Build history of the part. All positions in model axes, mm. Round coordinates to 2 decimals unless told otherwise and drop trailing zeros. Loops run counter-clockwise (first coordinate to the right, second up) from the corner with the lowest first, then second, coordinate; pieces in that order, holes last. Notation, with made-up numbers: (-32.5, 81.5) -> (-14.5, 81.5) arc R22 cw to (-14.5, 104.5) -> close; hole circle Ø7 at (-13.75, 78.25). An arc over 180 degrees is marked (long way). Put each result on its own line as item: value. Start each with the question number.
Item 1: Cut at A-A, the plane y = 4.5. List the corners of the cut face in (x, z).
Item 2: Cut at B-B, the plane z = 0. List the corners of the cut face in (x, y), plus the area to 3 significant figures.
Item 3: Drill centre lines: probe 1 along Z at (x, y) = (-2.5, 3.75); probe 2 along Z at (x, y) = (0, 2.5); probe 3 along X at (y, z) = (6.5, 1). Where is each one in solid material? Low to high. Write a range as [from, to].
Item 4: Cut at C-C, the plane x = 0. List the corners of the cut face in (y, z).
Item 5: Flat gauge pins, fed straight in: pin 1 Ø5.5 at (x, z) = (0, 0) entering from +Y; pin 2 Ø3 at (x, y) = (-1, 4) entering from +Z; pin 3 Ø3 at (x, y) = (-24, 1.5) entering from +Z; pin 4 Ø1 at (x, y) = (29, 7) entering from -Z. Where does each tip first touch, or does it go through?
Item 6: Pull direction Z, two halves, no side cores. Call faces 1 (the cylindrical face through (-1.73, 5.22, -7.81)), 2 (the flat face through (-1, 8, 9)), 3 (the conical face through (27.85, 0.14, -28.21)), 4 (the flat face through (3.4, 3, -3.4)): +Z half, -Z half, draft (parallel to the pull), parting line (faces both ways), or undercut.
```python
from build123d import *

# Parameters (mm, degrees)
F0_R     = 8
F1_DEPTH = 8
F0_R_2   = 4.5
F2_DEPTH = 3
F3_SIZE  = 0.5
F4_SIZE  = 2


with BuildPart() as f1:
    # F0 (on Front) → F1 (new body)
    with BuildSketch(Plane.XZ):
        with BuildLine():
            Line((-7.7551369733, 32.692779792), (-12.9187443003, 37.856387119))
            ThreePointArc((-12.9187443003, 37.856387119), (-28.2842712475, 28.2842712475), (-37.856387119, 12.9187443003))
            Line((-37.856387119, 12.9187443003), (-32.692779792, 7.7551369733))
            ThreePointArc((-32.692779792, 7.7551369733), (-23.7587878479, 23.7587878479), (-7.7551369733, 32.692779792))
        make_face()
        with BuildLine():
            Line((-5.0414182424, 29.9790610611), (-7.7551369733, 32.692779792))
            ThreePointArc((-7.7551369733, 32.692779792), (-23.7587878479, 23.7587878479), (-32.692779792, 7.7551369733))
            Line((-32.692779792, 7.7551369733), (-29.9790610611, 5.0414182424))
            ThreePointArc((-29.9790610611, 5.0414182424), (-29.423423687, 7.6434376124), (-28.6423974084, 10.1869068269))
            ThreePointArc((-28.6423974084, 10.1869068269), (-29.5179510637, 12.2267356641), (-27.4564643335, 13.0500025402))
            ThreePointArc((-27.4564643335, 13.0500025402), (-25.276676214, 16.8893350838), (-22.5637642579, 20.3724456684))
            ThreePointArc((-22.5637642579, 20.3724456684), (-22.5920616589, 22.5920616589), (-20.3724456684, 22.5637642579))
            ThreePointArc((-20.3724456684, 22.5637642579), (-16.8893350838, 25.276676214), (-13.0500025402, 27.4564643335))
            ThreePointArc((-13.0500025402, 27.4564643335), (-12.2267356641, 29.5179510637), (-10.1869068269, 28.6423974084))
            ThreePointArc((-10.1869068269, 28.6423974084), (-7.6434376124, 29.423423687), (-5.0414182424, 29.9790610611))
        make_face()
        with BuildLine():
            Line((-0.0622796062, 24.9999224249), (-5.0414182424, 29.9790610611))
            ThreePointArc((-5.0414182424, 29.9790610611), (-7.6434376124, 29.423423687), (-10.1869068269, 28.6423974084))
            ThreePointArc((-10.1869068269, 28.6423974084), (-10.1096278948, 28.3689238734), (-10.0835763439, 28.0859377883))
            ThreePointArc((-10.0835763439, 28.0859377883), (-11.3118315726, 26.5696989212), (-13.0500025402, 27.4564643335))
            ThreePointArc((-13.0500025402, 27.4564643335), (-16.8893350838, 25.276676214), (-20.3724456684, 22.5637642579))
            ThreePointArc((-20.3724456684, 22.5637642579), (-20.0565877875, 22.0709023286), (-19.9460461481, 21.4960461481))
            ThreePointArc((-19.9460461481, 21.4960461481), (-20.8846800835, 20.0717106767), (-22.5637642579, 20.3724456684))
            ThreePointArc((-22.5637642579, 20.3724456684), (-25.276676214, 16.8893350838), (-27.4564643335, 13.0500025402))
            ThreePointArc((-27.4564643335, 13.0500025402), (-26.7862870939, 12.4782112192), (-26.5359377883, 11.6335763439))
            ThreePointArc((-26.5359377883, 11.6335763439), (-27.2084448855, 10.3558806816), (-28.6423974084, 10.1869068269))
            ThreePointArc((-28.6423974084, 10.1869068269), (-29.423423687, 7.6434376124), (-29.9790610611, 5.0414182424))
            Line((-29.9790610611, 5.0414182424), (-24.9999224249, 0.0622796062))
            ThreePointArc((-24.9999224249, 0.0622796062), (-17.6776695297, 17.6776695297), (-0.0622796062, 24.9999224249))
        make_face()
        with BuildLine():
            Line((24.9999224249, -0.0622796062), (-0.0622796062, 24.9999224249))
            ThreePointArc((-0.0622796062, 24.9999224249), (-17.6776695297, 17.6776695297), (-24.9999224249, 0.0622796062))
            Line((-24.9999224249, 0.0622796062), (0.0622796062, -24.9999224249))
            ThreePointArc((0.0622796062, -24.9999224249), (17.6776695297, -17.6776695297), (24.9999224249, -0.0622796062))
        make_face()
        Circle(F0_R, mode=Mode.SUBTRACT)
        with BuildLine():
            ThreePointArc((28.6423974084, -10.1869068269), (29.423423687, -7.6434376124), (29.9790610611, -5.0414182424))
            Line((29.9790610611, -5.0414182424), (24.9999224249, -0.0622796062))
            ThreePointArc((24.9999224249, -0.0622796062), (17.6776695297, -17.6776695297), (0.0622796062, -24.9999224249))
            Line((0.0622796062, -24.9999224249), (5.0414182424, -29.9790610611))
            ThreePointArc((5.0414182424, -29.9790610611), (7.6434376124, -29.423423687), (10.1869068269, -28.6423974084))
            ThreePointArc((10.1869068269, -28.6423974084), (11.0404170237, -26.653924513), (13.0500025402, -27.4564643335))
            ThreePointArc((13.0500025402, -27.4564643335), (16.8893350838, -25.276676214), (20.3724456684, -22.5637642579))
            ThreePointArc((20.3724456684, -22.5637642579), (20.4000306372, -20.4000306372), (22.5637642579, -20.3724456684))
            ThreePointArc((22.5637642579, -20.3724456684), (25.276676214, -16.8893350838), (27.4564643335, -13.0500025402))
            ThreePointArc((27.4564643335, -13.0500025402), (26.653924513, -11.0404170237), (28.6423974084, -10.1869068269))
        make_face()
        with BuildLine():
            ThreePointArc((7.7551369733, -32.692779792), (23.7587878479, -23.7587878479), (32.692779792, -7.7551369733))
            Line((32.692779792, -7.7551369733), (29.9790610611, -5.0414182424))
            ThreePointArc((29.9790610611, -5.0414182424), (29.423423687, -7.6434376124), (28.6423974084, -10.1869068269))
            ThreePointArc((28.6423974084, -10.1869068269), (29.3636334507, -10.7560834411), (29.6359377883, -11.6335763439))
            ThreePointArc((29.6359377883, -11.6335763439), (28.9305726636, -12.9332270383), (27.4564643335, -13.0500025402))
            ThreePointArc((27.4564643335, -13.0500025402), (25.276676214, -16.8893350838), (22.5637642579, -20.3724456684))
            ThreePointArc((22.5637642579, -20.3724456684), (22.9203816195, -20.8846800835), (23.0460461481, -21.4960461481))
            ThreePointArc((23.0460461481, -21.4960461481), (22.0709023286, -22.9355045086), (20.3724456684, -22.5637642579))
            ThreePointArc((20.3724456684, -22.5637642579), (16.8893350838, -25.276676214), (13.0500025402, -27.4564643335))
            ThreePointArc((13.0500025402, -27.4564643335), (13.149815211, -27.7641930171), (13.1835763439, -28.0859377883))
            ThreePointArc((13.1835763439, -28.0859377883), (11.916562429, -29.6098862375), (10.1869068269, -28.6423974084))
            ThreePointArc((10.1869068269, -28.6423974084), (7.6434376124, -29.423423687), (5.0414182424, -29.9790610611))
            Line((5.0414182424, -29.9790610611), (7.7551369733, -32.692779792))
        make_face()
        with BuildLine():
            ThreePointArc((12.9187443003, -37.856387119), (28.2842712475, -28.2842712475), (37.856387119, -12.9187443003))
            Line((37.856387119, -12.9187443003), (32.692779792, -7.7551369733))
            ThreePointArc((32.692779792, -7.7551369733), (23.7587878479, -23.7587878479), (7.7551369733, -32.692779792))
            Line((7.7551369733, -32.692779792), (12.9187443003, -37.856387119))
        make_face()
    extrude(amount=-F1_DEPTH)

    # F0 (on Front) → F2 (join)
    with BuildSketch(Plane.XZ):
        Circle(F0_R)
        Circle(F0_R_2, mode=Mode.SUBTRACT)
    extrude(amount=-F2_DEPTH)

    # F3
    f3_edges = [f1.edges().sort_by_distance(p)[0] for p in [
        (-28.284271, 8, 28.284271),
        (-12.468821, 8, -12.468821),
        (28.284271, 8, -28.284271),
        (12.468821, 8, 12.468821),
        (10.21715, 8, -28.715411),
        (20.428328, 8, -22.619647),
        (27.529478, 8, -13.080246),
        (-28.715411, 8, 10.21715),
        (-22.619647, 8, 20.428328),
        (-13.080246, 8, 27.529478),
        (-8, 8, 0),
        (-4.5, 0, 0),
        (12.468821, 0, 12.468821),
        (-28.284271, 0, 28.284271),
        (-12.468821, 0, -12.468821),
        (28.284271, 0, -28.284271),
    ]]
    chamfer(f3_edges, length=F3_SIZE)

    # F4
    f4_edges = [f1.edges().sort_by_distance(p)[0] for p in [
        (-28.715411, 0, 10.21715),
        (-22.619647, 0, 20.428328),
        (-13.080246, 0, 27.529478),
        (27.529478, 0, -13.080246),
        (20.428328, 0, -22.619647),
        (10.21715, 0, -28.715411),
    ]]
    chamfer(f4_edges, length=F4_SIZE)


solid = f1.part
```
Reply:
1. outline: (-37.86, 12.92) -> (12.92, -37.86) arc R40 ccw to (37.86, -12.92) -> (-12.92, 37.86) arc R40 ccw to start; hole circle Ø3.1 at (-28.09, 11.63); hole circle Ø3.1 at (-21.5, 21.5); hole circle Ø3.1 at (-11.63, 28.09); hole circle Ø16 at (0, 0); hole circle Ø3.1 at (11.63, -28.09); hole circle Ø3.1 at (21.5, -21.5); hole circle Ø3.1 at (28.09, -11.63)
2. outline: (-24.94, 0.5) -> (-24.23, 0) -> (-5, 0) -> (-4.5, 0.5) -> (-4.5, 3) -> (-8, 3) -> (-8, 7.5) -> (-8.5, 8) -> (-24.23, 8) -> (-24.94, 7.5) -> close; (4.5, 0.5) -> (5, 0) -> (24.23, 0) -> (24.94, 0.5) -> (24.94, 7.5) -> (24.23, 8) -> (8.5, 8) -> (8, 7.5) -> (8, 3) -> (4.5, 3) -> close
2. area: 291 mm^2
3. probe 1: z = [-22.44, -7.6], [7.6, 27.44]
3. probe 2: z = [-24.94, -4.5], [4.5, 24.94]
3. probe 3: x = [-25.94, -7.94], [7.94, 23.94]
4. outline: (0, -24.23) -> (0.5, -24.94) -> (7.5, -24.94) -> (8, -24.23) -> (8, -8.5) -> (7.5, -8) -> (3, -8) -> (3, -4.5) -> (0.5, -4.5) -> (0, -5) -> close; (0, 5) -> (0.5, 4.5) -> (3, 4.5) -> (3, 8) -> (7.5, 8) -> (8, 8.5) -> (8, 24.23) -> (7.5, 24.94) -> (0.5, 24.94) -> (0, 24.23) -> close
5. pin 1: passes through
5. pin 2: stops at z = 27.44
5. pin 3: stops at z = 33.07
5. pin 4: stops at z = -28.07
6. face 1: undercut
6. face 2: draft
6. face 3: -Z half
6. face 4: undercut
